Geometry: final body of the model. Coordinates: model frame, mm. Face numbers are marked on the shaded views. A direction names the side the tool comes from. Coordinates: 2 decimals unless noted, no trailing zeros. Loops run counter-clockwise (first coordinate to the right, second up) from the corner with the lowest first, then second, coordinate; pieces in that order, holes last. Notation, with made-up numbers: (13, 69) -> (66, 69) arc R21 ccw to (66, 83) -> close; hole circle Ø6 at (19.5, 65). An arc over 180 degrees is marked (long way). One line per item, written item: value. Start each with the question number.
Item 1: Section query C-C on z = 22.5. Return loops of the section in (x, y), then the cut area to 3 significant figures.
Item 2: Contact query for flat-ended pins moving along their axis: pin 1 Ø1 at (x, y) = (-0.5, 0) entering from +Z; pin 2 Ø2 at (y, z) = (1, 14) entering from +X; pin 3 Ø2 at (x, z) = (4.5, 20.5) entering from -Y. Output: stop coordinate, or through.
Item 3: Set-up query: the marked faces 1 and 2. Return all of +Z, -Z, +X, -X, +Y, -Y with unobstructed straight access to the full face (end or side cutting, diameter ignored); none if empty.
Item 4: Section query A-A on x = 0. Return loops of the section in (y, z), then the cut area to 3 significant figures.
Item 5: Ray query, probe 1 along Y at (x, z) = (0, 18.5); probe 2 along X at (y, z) = (0.5, 5.5); probe 3 along X at (y, z) = (1.5, 11.5). Return the intervals inside material, ascending. Write a range as from..to.
from build123d import *

# Parameters (mm, degrees)
F0_R     = 5.75
F1_DEPTH = 30
F2_R     = 1.75
F3_DEPTH = 25
F4_R     = 1


with BuildPart() as f1:
    # F0 (on Top) → F1 (new body)
    with BuildSketch(Plane.XY):
        Circle(F0_R)
    extrude(amount=F1_DEPTH)

    # F2 (on face) → F3 (cut)
    with BuildSketch(Plane.XY.offset(30)):
        Circle(F2_R)
    extrude(amount=-F3_DEPTH, mode=Mode.SUBTRACT)

    # F4
    f4_edges = [f1.edges().sort_by_distance(p)[0] for p in [
        (-5.75, 0, 30),
    ]]
    fillet(f4_edges, radius=F4_R)


solid = f1.part
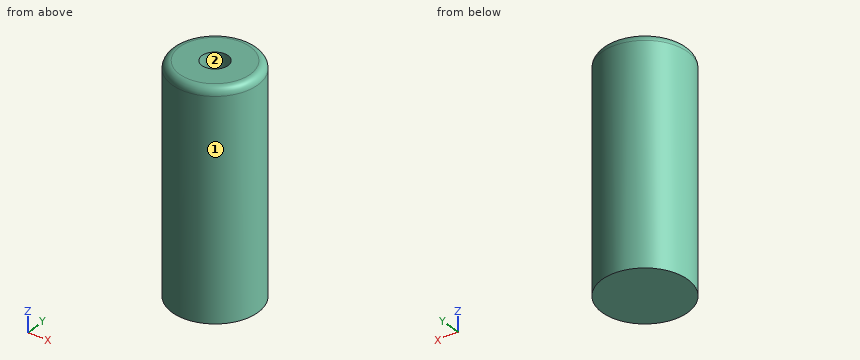
Reply:
1. outline: circle Ø11.5 at (0, 0); hole circle Ø3.5 at (0, 0)
1. area: 94.2 mm²
2. pin 1: stops at z = 5
2. pin 2: stops at x = 5.75
2. pin 3: stops at y = -4.56
3. face 1: +Z, -Z
3. face 2: +Z
4. outline: (-5.75, 0) -> (5.75, 0) -> (5.75, 29) arc R1 ccw to (4.75, 30) -> (1.75, 30) -> (1.75, 5) -> (-1.75, 5) -> (-1.75, 30) -> (-4.75, 30) arc R1 ccw to (-5.75, 29) -> close
4. area: 257 mm²
5. probe 1: y = -5.75..-1.75, 1.75..5.75
5. probe 2: x = -5.73..-1.68, 1.68..5.73
5. probe 3: x = -5.55..-0.9, 0.9..5.55
